Job drawing, mm, ordinate dimensions from the low corner. One solid piece. A direction names the side the tool comes from. Round coordinates to 2 decimals unless told otherwise and drop trailing zeros. Loops run counter-clockwise (first coordinate to the right, second up) from the corner with the lowest first, then second, coordinate; pieces in that order, holes last.
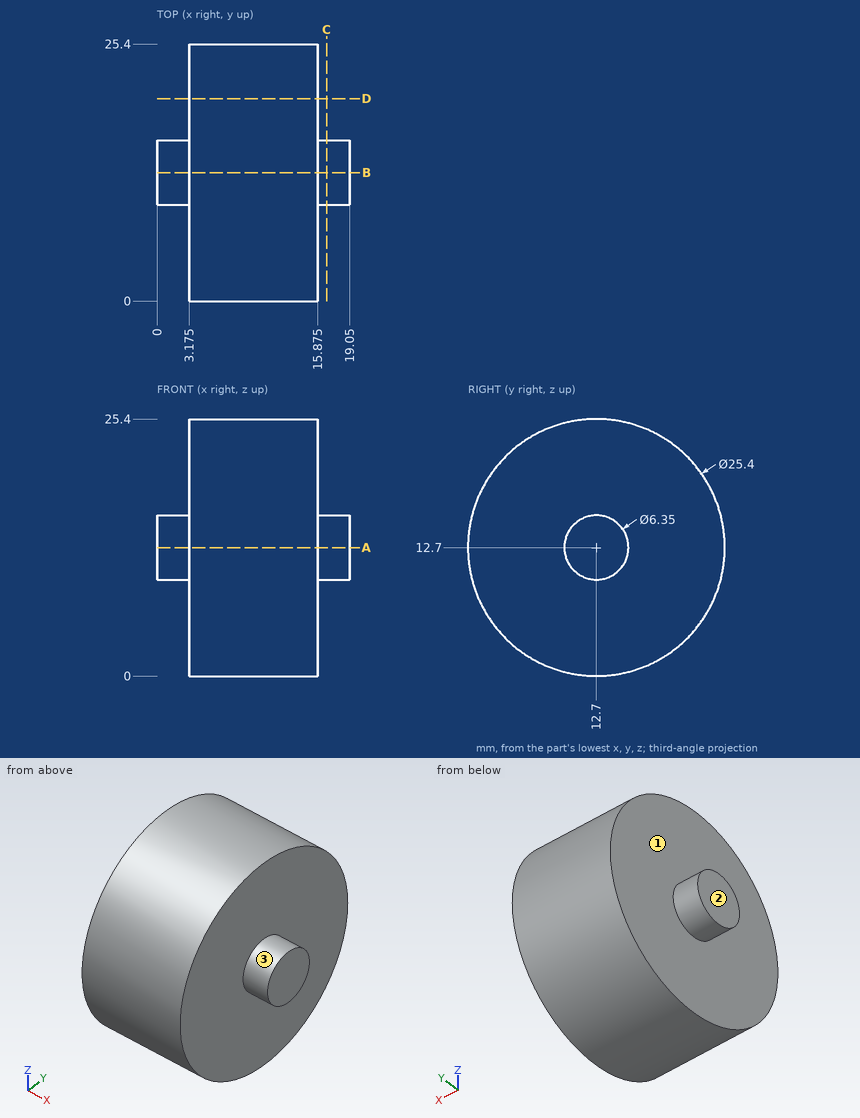
1) Slice it at C-C, the plane x = 16.75. Give the cut face in (y, z) (3 decimals).
Values:
outline: circle Ø6.35 at (12.7, 12.7)
2) Drop flat-ended pins along their axis: pin 1 Ø8 at (x, z) = (6, 22) entering from -Y; pin 2 Ø1 at (x, z) = (10, 5.5) entering from -Y; pin 3 Ø2 at (x, y) = (8.5, 7) entering from +Z. Give the stop position or say it passes through.
Values:
pin 1: stops at y = 1.16
pin 2: stops at y = 1.91
pin 3: stops at z = 24.5
3) Tool access for the marked faces 1, 2 and 3: list every direction of +Z, -Z, +X, -X, +Y, -Y with a clear straight run to the whole face (end or side of a thin tool).
Values:
face 1: -X
face 2: +Z, -Z, -X, +Y, -Y
face 3: +X
4) Wall check: line 1 along X through (y, z) = (16.5, 7) (3 decimals); line 2 along Y through (x, z) = (5, 13); line 3 along Y through (x, z) = (14.5, 20). Give the ranges that are in metal, low to high.
Values:
line 1: x = 3.175 to 15.875
line 2: y = 0 to 25.4
line 3: y = 2.31 to 23.09
5) Slice it at A-A, the plane z = 12.7. Give the cut face in (x, y) (3 decimals), then the cut area to 3 significant figures.
Values:
outline: (0, 9.525) - (3.175, 9.525) - (3.175, 0) - (15.875, 0) - (15.875, 9.525) - (19.05, 9.525) - (19.05, 15.875) - (15.875, 15.875) - (15.875, 25.4) - (3.175, 25.4) - (3.175, 15.875) - (0, 15.875) - close
area: 363 mm2
6) Slice it at D-D, the plane y = 20. Give the cut face in (x, z) (3 decimals).
Values:
outline: (3.175, 2.308) - (15.875, 2.308) - (15.875, 23.092) - (3.175, 23.092) - close
